Read the model definition and answer for the solid it produces. Units are mm, in the model's axes. A direction names the side the tool comes from. Coordinates: 2 decimals unless noted, no trailing zeros. Loops run counter-clockwise (first coordinate to the right, second up) from the corner with the lowest first, then second, coordinate; pieces in that order, holes last. Notation, with made-up numbers: (-13.5, 56.25) -> (30.5, 56.25) arc R24 cw to (30.5, 89.25) -> close; hole circle Ø6 at (-0.75, 15.5). An arc over 180 degrees is marked (long way). Answer as a JSON object with one key per item and string values. Group by question number.
Q1. Determine the mould class of faces 5 (the flat face through (-36, -52.351, -4)), 6 (the flat face through (-25, -31.636, -4)), 7 (the flat face through (-47.523, -43, -4)) for opening direction X: released by +X, released by -X, zero draft, split by the parting line, or undercut.
Q2. The part is cut by section A-A on x = -33.25. Write down the section's boundary in (y, z).
Q3. The part is cut by section C-C on y = -41.75. Write down the section's boundary in (x, z), and give its area (3 significant figures).
Q4. The part is cut by section D-D on x = -25.25. Write down the section's boundary in (y, z).
Q5. Each of these flat-tipped pins is pushed along its axis until it touches: P1, Ø7.5, axis at x = -38, z = -6, coming from the +Y side; P2, Ø3, axis at x = -37.5, y = -36, coming from the -Z side; P3, Ø2, axis at y = -53, z = -1.5, coming from the +X side; P4, Ø6, axis at y = -48.5, z = -10, coming from the +X side. Where does it stop, or does it pass through?
Q6. Straight lines are drawn through the part: line 1 along Y through (x, z) = (-36.75, -4.25); line 2 along X through (y, z) = (-37.75, -1.5); line 3 along Y through (x, z) = (-25.5, -4.5). For each, find the intervals that lie inside material, in ascending order. Write a range as [from, to].
Q7. For faces 1 (the flat face through (-26.023, -53, -4)), 2 (the flat face through (-37, -31.536, -4)), 3 (the flat face through (-36, -34, 3.068)), 4 (the flat face through (-35, -34.351, -4)), determine the directions among +Z, -Z, +X, -X, +Y, -Y from which every point of the face is accessible in a straight line to the end or side of a thin tool.
Autodesk Inventor part; units mm, degrees
ref_plane "YZ Plane" through (0, 0, 0) normal (1, 0, 0) x (0, 1, 0)
ref_plane "XZ Plane" through (0, 0, 0) normal (0, 1, 0) x (-1, 0, 0)
ref_plane "XY Plane" through (0, 0, 0) normal (0, 0, 1) x (1, 0, 0)
ref_plane "РабПлоскость3" through (-23.0229, -31.0507, 3.0679) normal (0, 0, 1) x (1, 0, 0)
sketch "Эскиз2" plane through (-23.0229, -31.0507, 3.0679) normal (0, 0, 1) x (1, 0, 0)
  arc A0 (-1, -3.4852) -> (-1, -0.4852) centre (0, -1.9852) ccw
  line L0 (-1, -3.4852) -> (-3, -3.4852)
  line L1 (-3, -0.4852) -> (-1, -0.4852)
  line L2 (-3, -0.4852) -> (-24.5, -0.4852)
  line L3 (-24.5, -0.4852) -> (-24.5, -3.2999)
  line L4 (-24.5, -3.2999) -> (-1.0821, -3.2999)
  line L5 (-3, -3.2999) -> (-3, -0.4852)
  line L6 (-24.5, -3.2999) -> (-22.5, -3.2999)
  line L7 (-22.5, -3.2999) -> (-22.5, -23.2999)
  line L8 (-22.5, -23.2999) -> (-24.5, -23.2999)
  line L9 (-24.5, -23.2999) -> (-24.5, -3.2999)
  line L10 (-22.5, -23.2999) -> (-3, -23.2999)
  line L11 (-3, -23.2999) -> (-3, -15.9662)
  line L12 (-3, -15.9662) -> (-22.5, -15.9662)
  line L13 (-22.5, -15.9662) -> (-22.5, -23.2999)
  line L14 (-1, -3.2999) -> (-22.5, -3.2999)
  line L15 (-22.5, -3.2999) -> (-22.5, -21.2999)
  line L16 (-3, -0.5852) -> (-0.9692, -0.5852)
  arc A1 (-1.0821, -3.2999) -> (-0.9692, -0.5852) centre (0, -1.9852) ccw
  line L17 (-0.9692, -3.3852) -> (-1.1358, -3.3852)
  line L18 (-1, -3.2999) -> (-22.5, -3.2999)
  line L19 (-22.5, -21.2999) -> (-1, -21.2999)
  point P0 (23.0229, 31.0507)
  point P1 (-22.5, -12.2999)
  point P2 (-3, -21.2999)
  point P3 (-22.5, -3.2999)
  point P4 (-3, -0.5852)
  dimension "d3" = 2
  dimension "d4" = 0.1
  dimension "d5" = 2
extrude "Выдавливание2" add sketch "Эскиз2" against normal blind 15 contours L5 L4 L3 L2 | L16 A1 L4 L5 | L4 L7 L8 L9 | L7 L19 L11 L10
properties part number "ЛЦМК.00002.00.00.00.00.22 Крышка короба"
Final values:
{
 "1": {"face 5": "zero draft", "face 6": "undercut", "face 7": "released by -X"},
 "2": {"outline": "(-54.35, -11.93) -> (-52.35, -11.93) -> (-52.35, 3.07) -> (-54.35, 3.07) -> close; (-34.35, -11.93) -> (-31.54, -11.93) -> (-31.54, 3.07) -> (-34.35, 3.07) -> close"},
 "3": {"outline": "(-47.52, -11.93) -> (-45.52, -11.93) -> (-45.52, 3.07) -> (-47.52, 3.07) -> close", "area": "30.0 mm2"},
 "4": {"outline": "(-34.35, -11.93) -> (-31.64, -11.93) -> (-31.64, 3.07) -> (-34.35, 3.07) -> close"},
 "5": {"P1": "stops at y = -31.54", "P2": "passes through", "P3": "stops at x = -26.02", "P4": "stops at x = -45.52"},
 "6": {"line 1": "y = [-54.35, -52.35], [-34.35, -31.54]", "line 2": "x = [-47.52, -45.52]", "line 3": "y = [-34.35, -31.64]"},
 "7": {"face 1": "+Z, -Z, +X, -Y", "face 2": "+Z, -Z, -X, +Y", "face 3": "+Z, +X, -X, +Y, -Y", "face 4": "+Z, -Z"}
}
